Check sheet for the drawn part. Datum: minimum x, y, z corner. Units: mm. A direction names the side the tool comes from. Give positions to 0.01 mm unless a question says otherwise; leave off trailing zeros. Write each loop counter-clockwise with the first axis right and the second up, starting at its lowest first coordinate (ties: lowest second). Pieces come first, ordered by that corner, then holes. Notation, with made-up numbers: M 14,14 L 24,14 A25 ccw 24,42 Z; hole C -18,25.25 d1. An arc over 180 degrees is marked long. Write item = value, one per line. Start each with the question number.
1) Set-up check for the marked faces 4 and 5: record each of +Z, -Z, +X, -X, +Y, -Y from which the full face is reachable in a straight line by a thin tool's end or side.
2) Draft check along X on the marked faces 1, 2 and 3. Enter one of: pulls with the +X half, pulls with the -X half, needs draft (parallel to the pull), parting line crosses it, or undercut.
3) Sectioned sample at B-B, the plane x = 54. Record the cut outline in (y, z).
4) Sectioned sample at A-A, the plane y = 14. Record the cut outline in (x, z), then the cut area to 3 significant figures.
5) Scan lines: L1, parallel to Z at x = 46, y = 31.5; L2, parallel to Y at x = 51, z = 34.5; L3, parallel to Z at x = 31.5, y = 5. Record each from-to range of solid material in increasing order.
6) Sectioned sample at D-D, the plane y = 37.5. Record the cut outline in (x, z).
7) Gauge pin test, flat ends, axial feed: pin 1 (3 mm diameter, centred on x = 20.5, z = 17.5, fed in from -Y); pin 2 (12 mm diameter, centred on y = 18, z = 12, fed in from -X); pin 3 (1.5 mm diameter, centred on x = 22, z = 32, fed in from +Y). Record the tip position at first contact, or that the pin passes through.
8) Sectioned sample at C-C, the plane z = 32. Record the cut outline in (x, y), then the cut area to 3 significant figures.
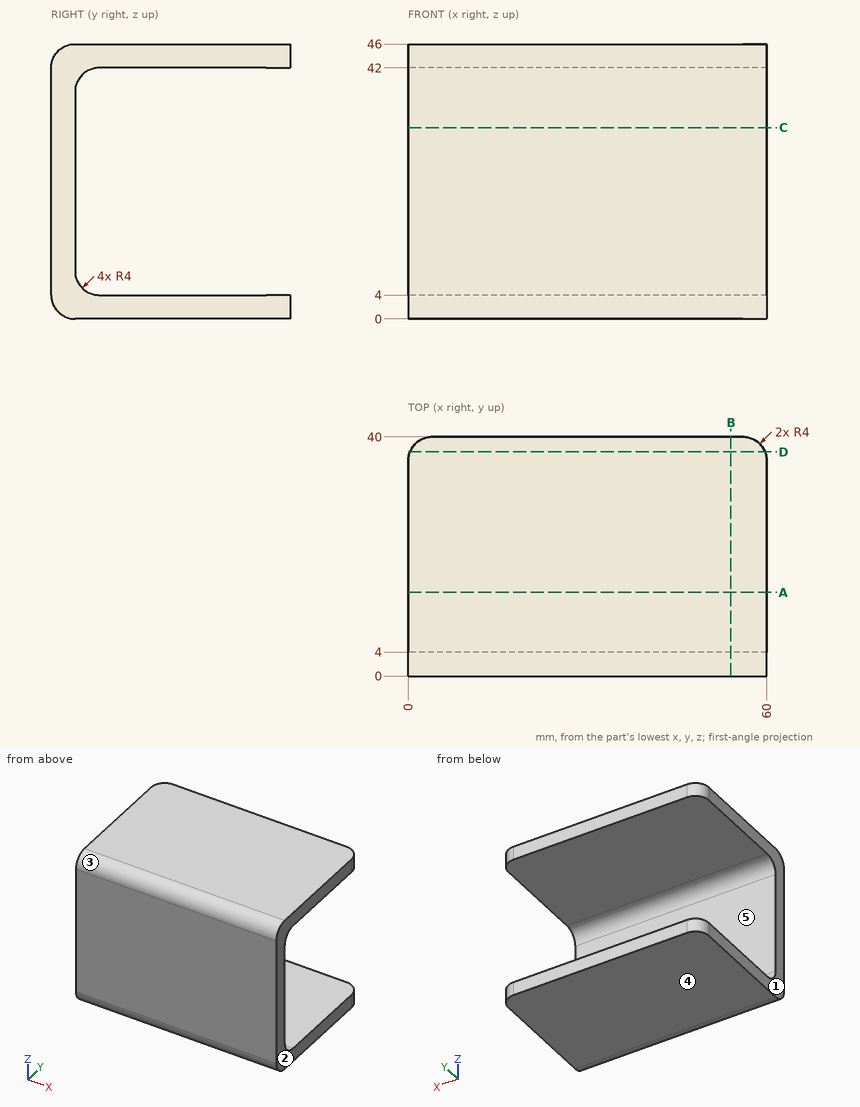
Data:
q1.face_4 = -Z, +X, -X, +Y, -Y
q1.face_5 = +X, -X, +Y
q2.face_1 = pulls with the -X half
q2.face_2 = pulls with the +X half
q2.face_3 = needs draft
q3.outline = M 0,4 A4 ccw 4,0 L 40,0 L 40,4 L 8,4 A4 cw 4,8 L 4,38 A4 cw 8,42 L 40,42 L 40,46 L 4,46 A4 ccw 0,42 Z
q4.outline = M 0,0 L 60,0 L 60,4 L 0,4 Z; M 0,42 L 60,42 L 60,46 L 0,46 Z
q4.area = 480 mm2
q5.L1 = 0 to 4, 42 to 46
q5.L2 = 0 to 4
q5.L3 = 0 to 5.35, 40.65 to 46
q6.outline = M 0.29,0 L 59.71,0 L 59.71,4 L 0.29,4 Z; M 0.29,42 L 59.71,42 L 59.71,46 L 0.29,46 Z
q7.pin_1 = 0
q7.pin_2 = through
q7.pin_3 = 4
q8.outline = M 0,0 L 60,0 L 60,4 L 0,4 Z
q8.area = 240 mm2
